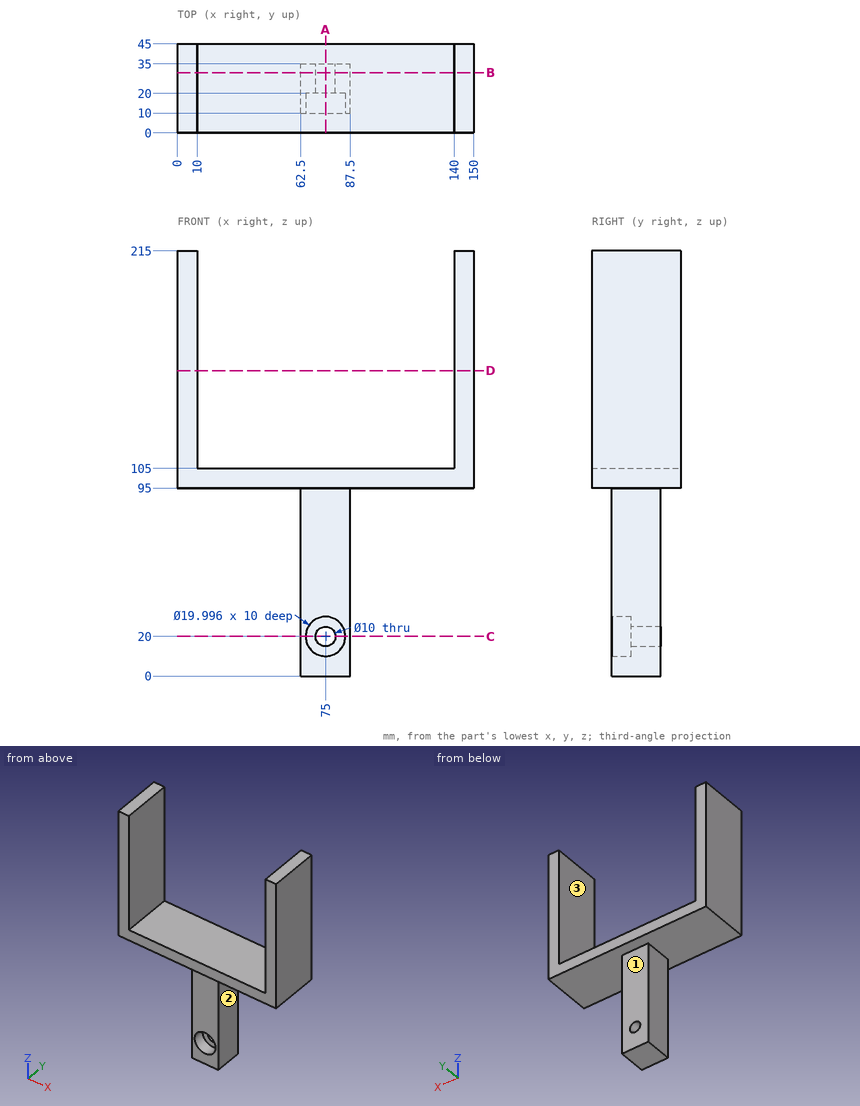
Check sheet for the drawn part. Datum: minimum x, y, z corner. Units: mm. A direction names the side the tool comes from. Coordinates: 2 decimals unless noted, no trailing zeros. Write each loop counter-clockwise with the first axis right and the second up, starting at its lowest first coordinate (ties: lowest second). Pieces come first, ordered by that corner, then holes. Notation, with made-up numbers: M 42.5,15.5 L 101.5,15.5 A25 ccw 101.5,29.5 Z; hole C 72.5,30.25 d3. An arc over 180 degrees is marked long. One line per item, written item: value.
Item 1: Gauge pin test, flat ends, axial feed: pin 1 Ø10 at (y, z) = (39, 111.5) entering from -X; pin 2 Ø7.5 at (x, z) = (78.5, 45.5) entering from -Y; pin 3 Ø12.5 at (x, z) = (71, 25.5) entering from +Y; pin 4 Ø12.5 at (y, z) = (23.5, 64.5) entering from +X. Record the tip position at first contact, or that the pin passes through.
Check sheet entries:
pin 1: stops at x = 0
pin 2: stops at y = 10
pin 3: stops at y = 35
pin 4: stops at x = 87.5
Item 2: Section check B-B, the plane y = 30.5. Record the boundary of the cut face in (x, z), plus the area to 3 significant figures.
Check sheet entries:
outline: M 0,95 L 62.5,95 L 62.5,0 L 87.5,0 L 87.5,95 L 150,95 L 150,215 L 140,215 L 140,105 L 10,105 L 10,215 L 0,215 Z; hole C 75,20 d10
area: 6,000 mm^2
Item 3: Section check D-D, the plane z = 154.5. Record the boundary of the cut face in (x, y).
Check sheet entries:
outline: M 0,0 L 10,0 L 10,45 L 0,45 Z; M 140,0 L 150,0 L 150,45 L 140,45 Z
Item 4: Section check C-C, the plane z = 20. Record the boundary of the cut face in (x, y).
Check sheet entries:
outline: M 62.5,10 L 65,10 L 65,20 L 70,20 L 70,35 L 62.5,35 Z; M 80,20 L 85,20 L 85,10 L 87.5,10 L 87.5,35 L 80,35 Z
Item 5: Scan lines: line 1 along X through (y, z) = (13.5, 206.5); line 2 along X through (y, z) = (31, 20); line 3 along Z through (x, y) = (38.5, 41). Record each from-to range of solid material in increasing order.
Check sheet entries:
line 1: x = 0 to 10, 140 to 150
line 2: x = 62.5 to 70, 80 to 87.5
line 3: z = 95 to 105
Item 6: Section check A-A, the plane x = 75. Record the boundary of the cut face in (y, z), plus the area to 3 significant figures.
Check sheet entries:
outline: M 0,95 L 10,95 L 10,30 L 20,30 L 20,25 L 35,25 L 35,95 L 45,95 L 45,105 L 0,105 Z; M 10,0 L 35,0 L 35,15 L 20,15 L 20,10 L 10,10 Z
area: 2,480 mm^2
Item 7: Access from +Z, -Z, +X, -X, +Y, -Y to the whole of each face (thin tool, end or side, straight path). Record for the marked faces 1, 2 and 3.
Check sheet entries:
face 1: -Z, +X, -X, +Y
face 2: -Z, +X, +Y, -Y
face 3: +Z, +Y, -Y
